from build123d import *

# Parameters (mm, degrees)
SKETCH1_W           = 23.0378
SKETCH1_H           = 9.144
BOSS_EXTRUDE1_DEPTH = 18.1
SKETCH2_W           = 31.9
SKETCH2_H           = 9.144
BOSS_EXTRUDE2_DEPTH = 1.8
SKETCH3_W           = 23.0378
SKETCH3_H           = 9.144
BOSS_EXTRUDE3_DEPTH = 2.5
SKETCH4_R           = 4.572
BOSS_EXTRUDE4_DEPTH = 5
SKETCH5_R           = 2.794
BOSS_EXTRUDE5_DEPTH = 4


with BuildPart() as part:
    # Sketch1 → Boss-Extrude1 (new body)
    with BuildSketch(Plane(origin=(0, 0, 0), x_dir=(1, 0, 0), z_dir=(0, 1, 0))):
        with Locations((11.5189, 4.572)):
            Rectangle(SKETCH1_W, SKETCH1_H)
    extrude(amount=-BOSS_EXTRUDE1_DEPTH)

    # Sketch2 → Boss-Extrude2 (add)
    with BuildSketch(Plane(origin=(0, 0, 0), x_dir=(1, 0, 0), z_dir=(0, 1, 0))):
        with Locations((11.929019777, 4.572)):
            Rectangle(SKETCH2_W, SKETCH2_H)
    extrude(amount=BOSS_EXTRUDE2_DEPTH)

    # Sketch3 → Boss-Extrude3 (add)
    with BuildSketch(Plane(origin=(0, 1.8, 0), x_dir=(1, 0, 0), z_dir=(0, 1, 0))):
        with Locations((11.5189, 4.572)):
            Rectangle(SKETCH3_W, SKETCH3_H)
    extrude(amount=BOSS_EXTRUDE3_DEPTH)

    # Sketch4 → Boss-Extrude4 (add)
    with BuildSketch(Plane(origin=(0, 4.3, 0), x_dir=(1, 0, 0), z_dir=(0, 1, 0))):
        with Locations(Location((18.4658, 4.572, 0), (0, 0, 270))):
            Circle(SKETCH4_R)
    extrude(amount=BOSS_EXTRUDE4_DEPTH)

    # Sketch5 → Boss-Extrude5 (add)
    with BuildSketch(Plane(origin=(0, 4.3, 0), x_dir=(1, 0, 0), z_dir=(0, 1, 0))):
        with Locations((13.3858, 4.572)):
            Circle(SKETCH5_R)
    extrude(amount=BOSS_EXTRUDE5_DEPTH)


solid = part.part
Can you work these out from the model? Positions are in its coordinate system, mm. A direction names the side the tool comes from. Round coordinates to 2 decimals unless told otherwise and drop trailing zeros. Loops run counter-clockwise (first coordinate to the right, second up) from the corner with the lowest first, then second, coordinate; pieces in that order, holes last. Notation, with made-up numbers: (29, -26) - (66, -26) arc R27 ccw to (66, -1) - close; hole circle Ø4 at (47, 26). An arc over 180 degrees is marked (long way). Use CSV: the item, a comma, the result in double quotes. Start each with the question number.
1) For faces 1 (the flat face through (25, 0, -5)), 2 (the flat face through (22, 4.3, -8)), 3 (the flat face through (22, 4.3, -1)), which set-ups out of +Z, -Z, +X, -X, +Y, -Y let a thin tool reach every point of the face, with its end or its side?
2) Please list where these lines run through material, in increasing order: probe 1 along X at (y, z) = (-3.25, -6.5); probe 2 along Y at (x, z) = (6.5, -7.5); probe 3 along Y at (x, z) = (25, -1.5). Write a range as [from, to].
3) If we section it at C-C on y = -14.5: Write out the boundary of the cut face in (x, z).
4) If we section it at B-B on z = -8.5: Write out the boundary of the cut face in (x, y).
5) We'd pull the mould along X, two halves only. Please class faces 4 (the flat face through (27.879, 1, -5)), 5 (the flat face through (-2, 0, -5)), 6 (the cylindrical face through (10.593, 6.272, -4.652)), 7 (the flat face through (0, 3, -5)): released by +X, released by -X, zero draft, split by the parting line, or undercut.
6) If we section it at D-D on x = -1.5: Write out the boundary of the cut face in (y, z), plus the area to 3 significant figures.
7) For pin 1 Ø3 at (y, z) = (3.5, -3) entering from +X; pin 2 Ø1.2 at (x, z) = (-3, -2.5) entering from -Y; pin 3 Ø4 at (x, z) = (26.5, -2.5) entering from +Y, each with a flat end and sliding along its axis, tell me the tip position at first contact or that it passes through.
8) If we section it at A-A on x = 22.5: Write out the boundary of the cut face in (y, z), plus the area to 3 significant figures.
Geometry results:
1,face 1,"+Z, -Z, +X, -Y"
1,face 2,"-Z, +X, +Y"
1,face 3,"+Z, +X, +Y"
2,probe 1,"x = [0, 23.04]"
2,probe 2,"y = [-18.1, 4.3]"
2,probe 3,"y = [0, 1.8]"
3,outline,"(0, -9.14) - (23.04, -9.14) - (23.04, 0) - (0, 0) - close"
4,outline,"(-4.02, 0) - (0, 0) - (0, -18.1) - (23.04, -18.1) - (23.04, 0) - (27.88, 0) - (27.88, 1.8) - (23.04, 1.8) - (23.04, 4.3) - (20.81, 4.3) - (20.81, 9.3) - (16.13, 9.3) - (16.13, 4.3) - (0, 4.3) - (0, 1.8) - (-4.02, 1.8) - close"
5,face 4,"released by +X"
5,face 5,"zero draft"
5,face 6,"undercut"
5,face 7,"released by -X"
6,outline,"(0, -9.14) - (1.8, -9.14) - (1.8, 0) - (0, 0) - close"
6,area,"16.5 mm2"
7,pin 1,"stops at x = 23.04"
7,pin 2,"stops at y = 0"
7,pin 3,"stops at y = 1.8"
8,outline,"(-18.1, -9.14) - (4.3, -9.14) - (4.3, -6.72) - (9.3, -6.72) - (9.3, -2.42) - (4.3, -2.42) - (4.3, 0) - (-18.1, 0) - close"
8,area,"226 mm2"
